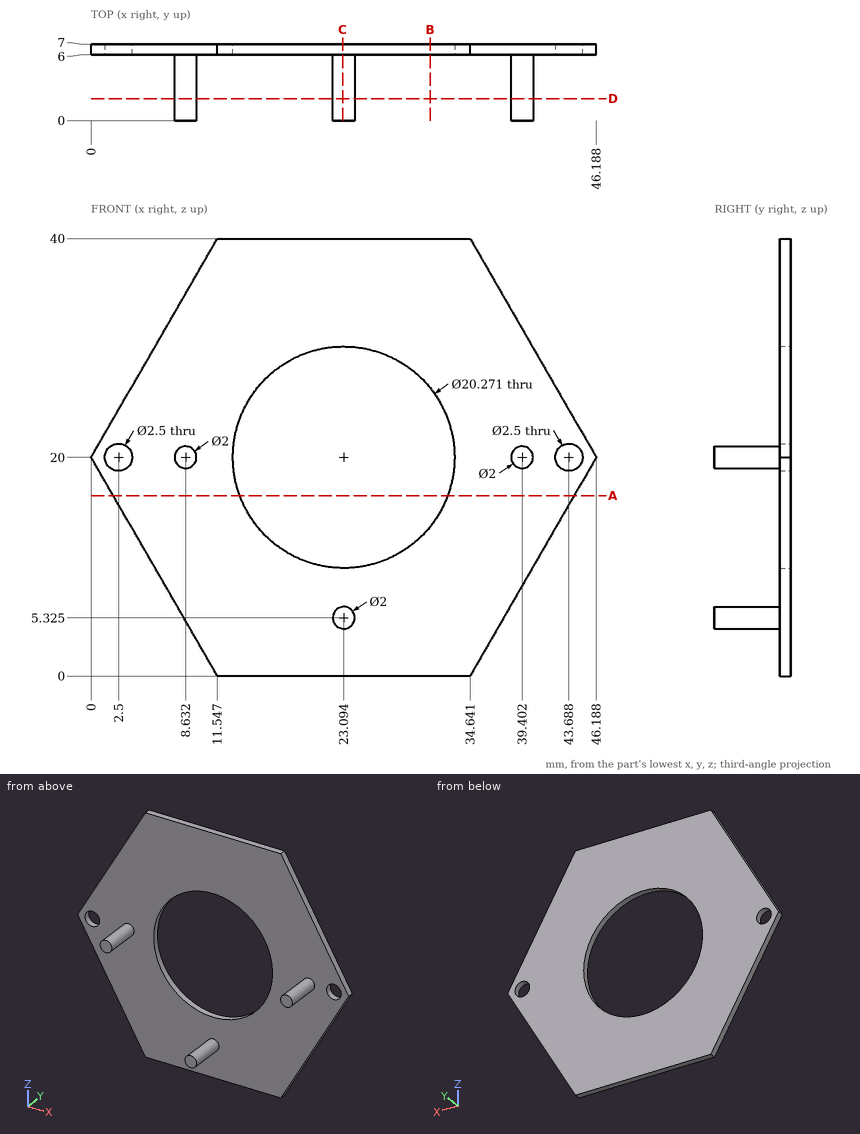
The drawing under review shows one solid part. Ordinate dimensions are in mm from its lowest x, y, z. Round coordinates to 2 decimals unless told otherwise and drop trailing zeros. Write each loop counter-clockwise with the first axis right and the second up, starting at its lowest first coordinate (ties: lowest second). Pieces come first, ordered by that corner, then holes. Notation, with made-up numbers: (39, -4.5) - (47, -4.5) arc R25 ccw to (47, 22.5) - close; hole circle Ø6 at (35.5, 80.25). An arc over 180 degrees is marked (long way). Use a Markdown table: item, result. Add a question column.
1. We need section D-D (y = 2). State the section outline as (x, z) points (1 decimal).
2. We need section B-B (x = 31). State the section outline as (y, z) points.
3. We need section A-A (z = 16.5). State the section outline as (x, y) points (1 decimal).
4. Wall thickness on probe 1 along Y at (x, z) = (32.5, 32); probe 2 along Z at (x, y) = (2.5, 6.6); probe 3 along Z at (x, y) = (28, 6.25): over which ranges is each line inside the solid? List them lowest first.
5. Clearance check with flat-ended pins moving along their axes: pin 1 (2 mm diameter, centred on x = 8, y = 6, fed in from +Z); pin 2 (2 mm diameter, centred on x = 2.5, z = 20, fed in from -Y); pin 3 (4 mm diameter, centred on y = 2.5, z = 20.5, fed in from +X); pin 4 (3 mm diameter, centred on x = 43.69, z = 20, fed in from -Y). State where each tip first meets the part, or that it passes through.
6. We need section C-C (x = 23). State the section outline as (y, z) points (1 decimal).
Output:
| question | item | result |
|---|---|---|
| 1 | outline | circle Ø2 at (8.6, 20); circle Ø2 at (23.1, 5.3); circle Ø2 at (39.4, 20) |
| 2 | outline | (6, 0) - (7, 0) - (7, 13.66) - (6, 13.66) - close; (6, 26.34) - (7, 26.34) - (7, 40) - (6, 40) - close |
| 3 | outline | (2, 6) - (13.6, 6) - (13.6, 7) - (2, 7) - close; (32.6, 6) - (44.2, 6) - (44.2, 7) - (32.6, 7) - close |
| 4 | probe 1 | y = 6 to 7 |
| 4 | probe 2 | z = 15.67 to 18.75, 21.25 to 24.33 |
| 4 | probe 3 | z = 0 to 11.13, 28.87 to 40 |
| 5 | pin 1 | stops at z = 35.59 |
| 5 | pin 2 | passes through |
| 5 | pin 3 | stops at x = 40.4 |
| 5 | pin 4 | stops at y = 6 |
| 6 | outline | (0, 4.3) - (6, 4.3) - (6, 0) - (7, 0) - (7, 9.9) - (6, 9.9) - (6, 6.3) - (0, 6.3) - close; (6, 30.1) - (7, 30.1) - (7, 40) - (6, 40) - close |
